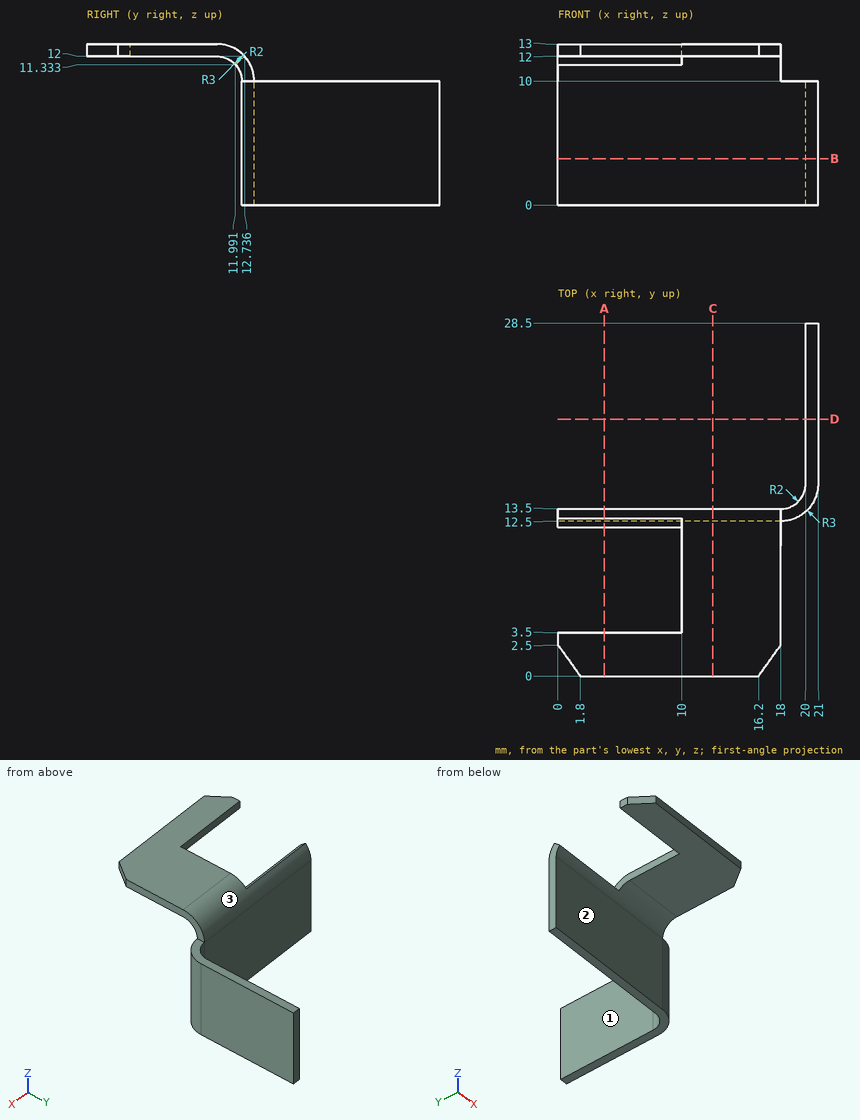
Here's the drawing with two shaded views (mm, measured from the low corner). I have some questions. A direction names the side the tool comes from. Coordinates: 2 decimals unless noted, no trailing zeros. Order: outer loops, then holes, each group sorted by start corner. A loop starts at its lowest first (then second) coordinate and runs counter-clockwise, first axis right, second up.
Item 1: If we section it at C-C on x = 12.5: List the corners of the cut face in (y, z) for me.
Result sheet:
outline: (0, 12) - (10.5, 12) arc R2 cw to (12.5, 10) - (12.5, 0) - (13.5, 0) - (13.5, 10) arc R3 ccw to (10.5, 13) - (0, 13) - close
Item 2: If we section it at A-A on x = 3.75: List the corners of the cut face in (y, z) for me, plus the area to 3 significant figures.
Result sheet:
outline: (0, 12) - (3.5, 12) - (3.5, 13) - (0, 13) - close; (11.99, 11.33) arc R2 cw to (12.5, 10) - (12.5, 0) - (13.5, 0) - (13.5, 10) arc R3 ccw to (12.74, 12) - close
area: 15.3 mm2
Item 3: If we section it at D-D on y = 20.75: List the corners of the cut face in (x, z) for me, plus the area to 3 significant figures.
Result sheet:
outline: (20, 0) - (21, 0) - (21, 10) - (20, 10) - close
area: 10.0 mm2
Item 4: For the marked faces 1, 2 and 3, which set-ups out of +Z, -Z, +X, -X, +Y, -Y let a thin tool reach every point of the face, with its end or its side?
Result sheet:
face 1: +Z, -Z, -X, +Y
face 2: -Z, +X, -X, -Y
face 3: +Z, +X, -X, +Y
Item 5: If we section it at B-B on z = 3.75: List the corners of the cut face in (x, y) for me.
Result sheet:
outline: (0, 12.5) - (18, 12.5) arc R3 ccw to (21, 15.5) - (21, 28.5) - (20, 28.5) - (20, 15.5) arc R2 cw to (18, 13.5) - (0, 13.5) - close
Item 6: For P1, Ø1.5, axis at x = 6, z = 7, coming from the -Y side; P2, Ø3.5, axis at y = 10, z = 12, coming from the +X side; P3, Ø4, axis at x = 17, y = 23.5, coming from the +Z side; P4, Ø8.5, axis at x = 13.5, y = 6.5, coming from the -Z side, each with a flat end and sliding along its axis, tell me the tip position at first contact or that it passes through.
Result sheet:
P1: stops at y = 12.5
P2: stops at x = 18
P3: passes through
P4: stops at z = 11.98
Item 7: I need wall thicknesses on line 1 (X direction, y = 24.5, z = 7); line 2 (Y direction, x = 6.75, z = 9); line 3 (Y direction, x = 18.75, z = 1.5) (1 decimal). Which ranges of each line are inside material? Lowest first, please.
Result sheet:
line 1: x = 20 to 21
line 2: y = 12.5 to 13.5
line 3: y = 12.6 to 13.6
